Check sheet for the modelled part. Datum: model origin and axes. Units: mm. Round coordinates to 2 decimals unless told otherwise and drop trailing zeros. Loops run counter-clockwise (first coordinate to the right, second up) from the corner with the lowest first, then second, coordinate; pieces in that order, holes last. Notation, with made-up numbers: (-36.75, 51) - (11.25, 51) arc R17 ccw to (11.25, 68) - close; hole circle Ø7 at (86.25, 8). An arc over 180 degrees is marked (long way). Return JSON: item names as keys, results as strings.
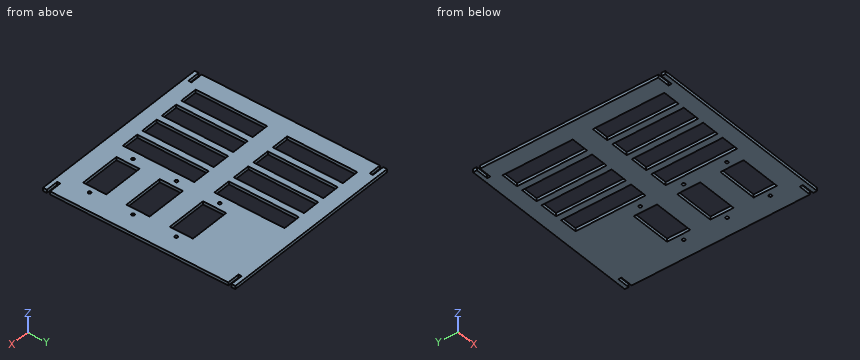
from build123d import *

# Parameters (mm, degrees)
SKETCH1_R           = 0.75
SKETCH1_W           = 20.574
SKETCH1_H           = 11.684
SKETCH1_W_2         = 8.89
SKETCH1_H_2         = 35.341542764
SKETCH1_H_3         = 36.036734061
BOSS_EXTRUDE1_DEPTH = 1.5875


with BuildPart() as part:
    # Sketch1 → Boss-Extrude1 (new body)
    with BuildSketch(Plane.XY):
        Polygon((0, 0), (93.98, 0), (93.98, 1.9685), (87.63, 1.9685), (87.63, 3.556), (93.98, 3.556), (93.98, 93.472), (87.63, 93.472), (87.63, 95.0595), (93.98, 95.0595), (93.98, 97.028), (0, 97.028), (0, 95.0595), (6.35, 95.0595), (6.35, 93.472), (0, 93.472), (0, 3.556), (6.35, 3.556), (6.35, 1.9685), (0, 1.9685), align=None)
        with Locations((57.807600894, 16.002)):
            Circle(SKETCH1_R, mode=Mode.SUBTRACT)
        with Locations((84.731600894, 16.002)):
            Circle(SKETCH1_R, mode=Mode.SUBTRACT)
        with Locations((57.807600894, 37.846)):
            Circle(SKETCH1_R, mode=Mode.SUBTRACT)
        with Locations((84.731600894, 37.846)):
            Circle(SKETCH1_R, mode=Mode.SUBTRACT)
        with Locations((57.807600894, 59.69)):
            Circle(SKETCH1_R, mode=Mode.SUBTRACT)
        with Locations((84.731600894, 59.69)):
            Circle(SKETCH1_R, mode=Mode.SUBTRACT)
        with Locations((71.269600894, 16.002)):
            Rectangle(SKETCH1_W, SKETCH1_H, mode=Mode.SUBTRACT)
        with Locations((71.269600894, 37.846)):
            Rectangle(SKETCH1_W, SKETCH1_H, mode=Mode.SUBTRACT)
        with Locations((71.269600894, 59.69)):
            Rectangle(SKETCH1_W, SKETCH1_H, mode=Mode.SUBTRACT)
        with Locations((25.290486919, 71.518771382)):
            Rectangle(SKETCH1_W_2, SKETCH1_H_2, mode=Mode.SUBTRACT)
        with Locations((13.225486919, 71.518771382)):
            Rectangle(SKETCH1_W_2, SKETCH1_H_2, mode=Mode.SUBTRACT)
        with Locations((13.225486919, 25.66963297)):
            Rectangle(SKETCH1_W_2, SKETCH1_H_3, mode=Mode.SUBTRACT)
        with Locations((25.290486919, 25.66963297)):
            Rectangle(SKETCH1_W_2, SKETCH1_H_3, mode=Mode.SUBTRACT)
        with Locations((37.355486919, 71.518771382)):
            Rectangle(SKETCH1_W_2, SKETCH1_H_2, mode=Mode.SUBTRACT)
        with Locations((37.355486919, 25.66963297)):
            Rectangle(SKETCH1_W_2, SKETCH1_H_3, mode=Mode.SUBTRACT)
        with Locations((49.420486919, 71.518771382)):
            Rectangle(SKETCH1_W_2, SKETCH1_H_2, mode=Mode.SUBTRACT)
        with Locations((49.420486919, 25.66963297)):
            Rectangle(SKETCH1_W_2, SKETCH1_H_3, mode=Mode.SUBTRACT)
    extrude(amount=BOSS_EXTRUDE1_DEPTH)


solid = part.part
Q1. Sectioned sample at A-A (y = 13.5). Enter the section's corners in (x, z), plus the area to 3 significant figures.
Answer key:
{"outline": "(0, 0) - (8.78, 0) - (8.78, 1.59) - (0, 1.59) - close; (17.67, 0) - (20.85, 0) - (20.85, 1.59) - (17.67, 1.59) - close; (29.74, 0) - (32.91, 0) - (32.91, 1.59) - (29.74, 1.59) - close; (41.8, 0) - (44.98, 0) - (44.98, 1.59) - (41.8, 1.59) - close; (53.87, 0) - (60.98, 0) - (60.98, 1.59) - (53.87, 1.59) - close; (81.56, 0) - (93.98, 0) - (93.98, 1.59) - (81.56, 1.59) - close", "area": "60.1 mm²"}
Q2. Sectioned sample at B-B (x = 46.5). Enter the section's corners in (y, z).
Answer key:
{"outline": "(0, 0) - (7.65, 0) - (7.65, 1.59) - (0, 1.59) - close; (43.69, 0) - (53.85, 0) - (53.85, 1.59) - (43.69, 1.59) - close; (89.19, 0) - (97.03, 0) - (97.03, 1.59) - (89.19, 1.59) - close"}
Q3. Sectioned sample at C-C (y = 85). Enter the section's corners in (x, z).
Answer key:
{"outline": "(0, 0) - (8.78, 0) - (8.78, 1.59) - (0, 1.59) - close; (17.67, 0) - (20.85, 0) - (20.85, 1.59) - (17.67, 1.59) - close; (29.74, 0) - (32.91, 0) - (32.91, 1.59) - (29.74, 1.59) - close; (41.8, 0) - (44.98, 0) - (44.98, 1.59) - (41.8, 1.59) - close; (53.87, 0) - (93.98, 0) - (93.98, 1.59) - (53.87, 1.59) - close"}
Q4. Scan lines: probe 1 along Y at (x, z) = (15, 1.3); probe 2 along X at (y, z) = (78.5, 1.2); probe 3 along X at (y, z) = (63, 0.5). Record each from-to range of solid material in increasing order. Write a range as [from, to].
Answer key:
{"probe 1": "y = [0, 7.65], [43.69, 53.85], [89.19, 97.03]", "probe 2": "x = [0, 8.78], [17.67, 20.85], [29.74, 32.91], [41.8, 44.98], [53.87, 93.98]", "probe 3": "x = [0, 8.78], [17.67, 20.85], [29.74, 32.91], [41.8, 44.98], [53.87, 60.98], [81.56, 93.98]"}
Q5. Sectioned sample at D-D (z = 0.45). State how many separate pieces and enclosed holes the cut face has, plus the area to 3 significant figures.
Answer key:
{"separate pieces": "1", "enclosed holes": "17", "area": "5,810 mm²"}
